The listing builds one solid part. Answer for the finished solid, in the listing's coordinates (mm). Face numbers are marked on the shaded views. A direction names the side the tool comes from. Give positions to 0.01 mm unless a question says otherwise; leave off trailing zeros. Loops run counter-clockwise (first coordinate to the right, second up) from the corner with the lowest first, then second, coordinate; pieces in that order, holes last. Notation, with made-up numbers: M 27,1.5 L 47,1.5 A22 cw 47,35.5 Z; hole C 34.25,-38.75 d7. An arc over 180 degrees is marked long. Use one line per item in the form item = value. Start each with the question number.
1. The mould has two halves that part along X. Classify the marked faces 1, 2, 3 and 4: released by +X, released by -X, zero draft, split by the parting line, or undercut.
2. Straight lines are drawn through the part: line 1 (Y direction, x = 2.5, z = -3); line 2 (X direction, y = 0.25, z = -3.5); line 3 (Z direction, x = 4.5, y = 0.5). For each, find the intervals that lie inside material, in ascending order. Write a range as from..to.
3. Each of these flat-tipped pins is pushed along its axis until it touches: pin 1 Ø1.1 at (x, z) = (3.5, -3) entering from -Y; pin 2 Ø3 at (x, z) = (3.5, -3.5) entering from +Y. Where does it stop, or does it pass through?
4. The part is cut by section A-A (z = -2.5). Write down the section's boundary in (x, y), and give its area (3 significant figures).
5. The part is cut by section C-C (x = 1.5). Write down the section's boundary in (y, z).
6. The part is cut by section B-B (y = 0.4). Write down the section's boundary in (x, z), and give its area (3 significant figures).
7. The part is cut by section D-D (y = 1.9). Write down the section's boundary in (x, z), and give its area (3 significant figures).
8. For the marked faces 5 and 6, determine the directions among +Z, -Z, +X, -X, +Y, -Y from which every point of the face is accessible in a straight line to the end or side of a thin tool.
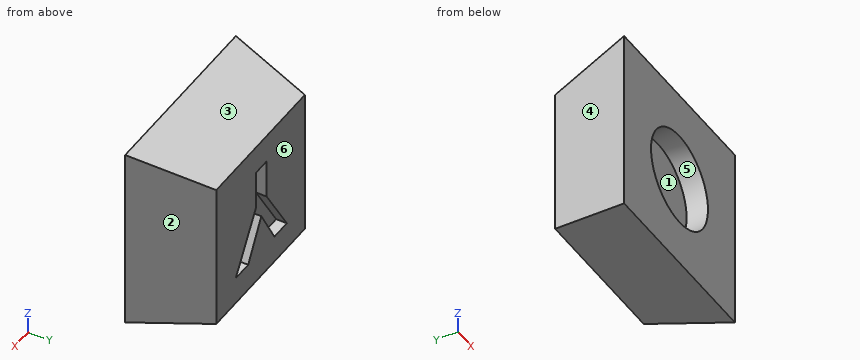
from build123d import *

# Parameters (mm, degrees)
SKETCH1_W           = 7
SKETCH1_H           = 7
BOSS_EXTRUDE1_DEPTH = 3
CUT_EXTRUDE1_DEPTH  = 7
CUT_EXTRUDE2_DEPTH  = 11
SKETCH4_R           = 1.8
CUT_EXTRUDE3_DEPTH  = 0.8
CUT_EXTRUDE4_DEPTH  = 0.4


with BuildPart() as part:
    # Sketch1 → Boss-Extrude1 (new body)
    with BuildSketch(Plane(origin=(0, 0, 0), x_dir=(1, 0, 0), z_dir=(0, 1, 0))):
        with Locations((3.5, 3.5)):
            Rectangle(SKETCH1_W, SKETCH1_H)
    extrude(amount=BOSS_EXTRUDE1_DEPTH)

    # Sketch2 → Cut-Extrude1 (cut)
    with BuildSketch(Plane.XY):
        Polygon((0, 0), (0.7, 3), (0, 3), align=None)
        Polygon((7, 0), (6.3, 3), (7, 3), align=None)
    extrude(amount=-CUT_EXTRUDE1_DEPTH, mode=Mode.SUBTRACT)

    # Sketch3 → Cut-Extrude2 (cut)
    with BuildSketch(Plane(origin=(0, 0, 0), x_dir=(0, 0, -1), z_dir=(1, 0, 0))):
        Polygon((0, 0), (0.7, 3), (0, 3), align=None)
        Polygon((7, 3), (6.3, 3), (7, 0), align=None)
    extrude(amount=CUT_EXTRUDE2_DEPTH, mode=Mode.SUBTRACT)

    # Sketch4 → Cut-Extrude3 (cut)
    with BuildSketch(Plane.XZ):
        with Locations(Location((3.5, -3.5, 0), (0, 0, 270))):
            Circle(SKETCH4_R)
    extrude(amount=-CUT_EXTRUDE3_DEPTH, mode=Mode.SUBTRACT)

    # Sketch5 → Cut-Extrude4 (cut)
    with BuildSketch(Plane(origin=(0, 3, 0), x_dir=(1, 0, 0), z_dir=(0, 1, 0))):
        Polygon((3.116897122, 1.759282352), (3.116897122, 3.232339243), (1.838050969, 5.259282352), (2.625410744, 5.259282352), (3.452734462, 3.81707482), (4.281460424, 5.259282352), (5.068820199, 5.259282352), (3.789974045, 3.22743139), (3.789974045, 1.759282352), align=None)
    extrude(amount=-CUT_EXTRUDE4_DEPTH, mode=Mode.SUBTRACT)


solid = part.part
Derived:
q1.face_1 = undercut
q1.face_2 = released by +X
q1.face_3 = zero draft
q1.face_4 = released by -X
q2.line_1 = 0.8..3
q2.line_2 = 0.06..1.7, 5.3..6.94
q2.line_3 = -6.88..-5, -2..-0.12
q3.pin_1 = 0.8
q3.pin_2 = 3
q4.outline = M 0,0 L 2,0 L 2,0.8 L 5,0.8 L 5,0 L 7,0 L 6.3,3 L 3.79,3 L 3.79,2.6 L 3.12,2.6 L 3.12,3 L 0.7,3 Z
q4.area = 16.2 mm2
q5.outline = M 0,-7 L 3,-6.3 L 3,-0.7 L 0,0 Z
q6.outline = M 0.09,-6.91 L 6.91,-6.91 L 6.91,-0.09 L 0.09,-0.09 Z; hole C 3.5,-3.5 d3.6
q6.area = 36.2 mm2
q7.outline = M 0.44,-6.56 L 6.56,-6.56 L 6.56,-0.44 L 0.44,-0.44 Z
q7.area = 37.4 mm2
q8.face_5 = -Y
q8.face_6 = +Z, -Z, +X, -X, +Y
